Verification items for this drawing (mm, ordinates from the low corner). A direction names the side the tool comes from. Give positions to 0.01 mm unless a question says otherwise; leave off trailing zeros. Loops run counter-clockwise (first coordinate to the right, second up) from the corner with the lowest first, then second, coordinate; pieces in that order, holes last. Notation, with made-up numbers: (14.5, 57) -> (72.5, 57) arc R4 cw to (72.5, 61) -> close; hole circle Ø8 at (-28, 39.25). An arc over 180 degrees is marked (long way). Answer in a Markdown table with one row per item. Add a question column.
Q1. Gauge pin test, flat ends, axial feed: P1, Ø6, axis at x = 5, z = 17.5, coming from the -Y side; P2, Ø5, axis at x = 4, z = 7.5, coming from the +Y side; P3, Ø5, axis at x = 2.5, z = 7.5, coming from the -Y side; P4, Ø6, axis at x = 8.5, z = 25, coming from the +Y side. Record the tip position at first contact, or that the pin passes through.
Q2. Section check A-A on y = 7. Enter the section's corners in (x, z), and give its area (3 significant figures).
Q3. Set-up check for the marked faces 1 and 2: record each of +Z, -Z, +X, -X, +Y, -Y from which the full face is reachable in a straight line by a thin tool's end or side.
Q4. Section check C-C on z = 28. Enter the section's corners in (x, y).
Q5. Material ranges on probe 1 along Y at (x, z) = (7, 0.7); probe 2 along Z at (x, y) = (11.5, 10); probe 3 along Y at (x, z) = (1.5, 5.5), recorded low to high.
Q6. Section check D-D on y = 9. Enter the section's corners in (x, z), and give its area (3 significant figures).
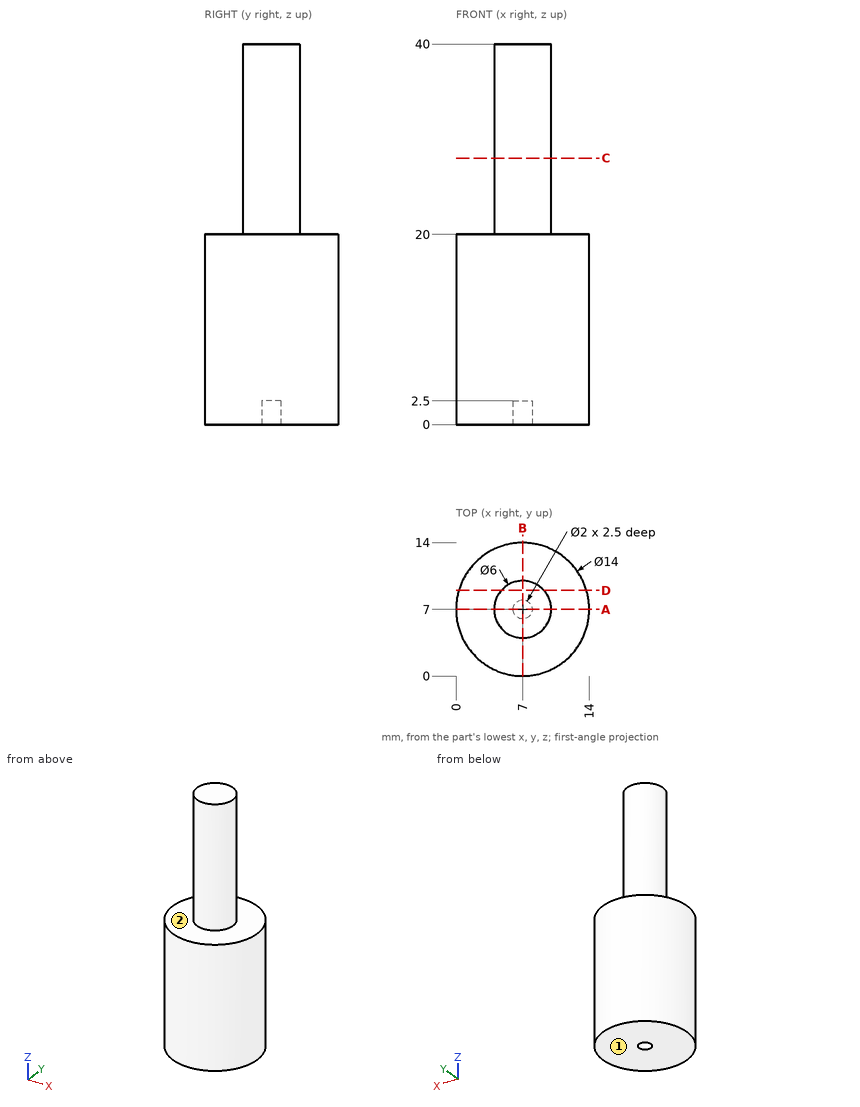
Taken from the geometry:
| question | item | result |
|---|---|---|
| 1 | P1 | stops at y = 0 |
| 1 | P2 | stops at y = 13.98 |
| 1 | P3 | stops at y = 0.29 |
| 1 | P4 | stops at y = 10 |
| 2 | outline | (0, 0) -> (6, 0) -> (6, 2.5) -> (8, 2.5) -> (8, 0) -> (14, 0) -> (14, 20) -> (10, 20) -> (10, 40) -> (4, 40) -> (4, 20) -> (0, 20) -> close |
| 2 | area | 395 mm² |
| 3 | face 1 | -Z, +X, -X, +Y, -Y |
| 3 | face 2 | +Z |
| 4 | outline | circle Ø6 at (7, 7) |
| 5 | probe 1 | y = 0 to 6, 8 to 14 |
| 5 | probe 2 | z = 0 to 20 |
| 5 | probe 3 | y = 2.67 to 11.33 |
| 6 | outline | (0.29, 0) -> (13.71, 0) -> (13.71, 20) -> (9.24, 20) -> (9.24, 40) -> (4.76, 40) -> (4.76, 20) -> (0.29, 20) -> close |
| 6 | area | 358 mm² |
